Part model, mm, in its own coordinate system. A direction names the side the tool comes from. Round coordinates to 2 decimals unless told otherwise and drop trailing zeros. Loops run counter-clockwise (first coordinate to the right, second up) from the corner with the lowest first, then second, coordinate; pieces in that order, holes last. Notation, with made-up numbers: M 52,22 L 110,22 A24 ccw 110,50 Z; hole C 65,41.25 d5. An arc over 180 degrees is marked long. Put each result on its own line as item: value. Start each with the question number.
```python
from build123d import *
from build123d.topology import SkipClean

# Parameters (mm, degrees)
ESQUISSE1_W                                       = 60.8
ESQUISSE1_H                                       = 121.6
BOSS_EXTRU_1_DEPTH                                = 91.2
ESQUISSE2_W                                       = 60.8
ESQUISSE2_H                                       = 60.8
ENL_V_MAT_EXTRU_1_DEPTH                           = 126.342411019
ESQUISSE3_W                                       = 51.8
ESQUISSE3_H                                       = 51.8
ENL_V_MAT_EXTRU_2_DEPTH                           = 60.8
BOSS_EXTRU_3_DEPTH                                = 4
ESQUISSE6_W                                       = 51.8
ESQUISSE6_H                                       = 51.8
ENL_V_MAT_EXTRU_3_DEPTH                           = 60.8
D_GAGEMENT_1_43_D                                 = 7.14248
FRAISAGE_POUR_VIS_T_TE_FRAIS_E_BOMB_E_D           = 4.3053
FRAISAGE_POUR_VIS_T_TE_FRAIS_E_BOMB_E_DEPTH       = 4.5
FRAISAGE_POUR_VIS_T_TE_FRAIS_E_BOMB_E_CSINK_D     = 7.0866
FRAISAGE_POUR_VIS_T_TE_FRAIS_E_BOMB_E_CSINK_ANGLE = 82
D_GAGEMENT_1_42_D                                 = 7.14248
D_GAGEMENT_1_42_DEPTH                             = 20
BOSS_EXTRU_5_DEPTH                                = 4
CHANFREIN1_SIZE                                   = 4
ESQUISSE26_W                                      = 60.8
ESQUISSE26_H                                      = 60.8
ESQUISSE26_W_2                                    = 51.800000032
ESQUISSE26_H_2                                    = 51.800000032
BOSS_EXTRU_8_DEPTH                                = 60.800000066
ESQUISSE27_R                                      = 3.57124
BOSS_EXTRU_9_DEPTH                                = 1.35


with BuildPart() as part:
    # Esquisse1 → Boss.-Extru.1 (new, symmetric)
    with BuildSketch(Plane.XY):
        Rectangle(ESQUISSE1_W, ESQUISSE1_H)
    extrude(amount=BOSS_EXTRU_1_DEPTH, both=True)

    # Esquisse2 → Enlèv. mat.-Extru.1 (cut, through all)
    with BuildSketch(Plane.ZY.offset(30.4)):
        with Locations((-60.8, 30.4)):
            Rectangle(ESQUISSE2_W, ESQUISSE2_H)
    enl_v_mat_extru_1 = extrude(amount=-ENL_V_MAT_EXTRU_1_DEPTH, mode=Mode.SUBTRACT)

    # Esquisse3 → Enlèv. mat.-Extru.2 (cut)
    with BuildSketch(Plane(origin=(0, 0, -91.2), x_dir=(-1, 0, 0), z_dir=(0, 0, -1))):
        with Locations((0, -30.4)):
            Rectangle(ESQUISSE3_W, ESQUISSE3_H)
    enl_v_mat_extru_2 = extrude(amount=-ENL_V_MAT_EXTRU_2_DEPTH, mode=Mode.SUBTRACT)

    # Symétrie2: Enlèv. mat.-Extru.1, Enlèv. mat.-Extru.2 across plane
    add(enl_v_mat_extru_1.mirror(Plane.XY), mode=Mode.SUBTRACT)
    add(enl_v_mat_extru_2.mirror(Plane.XY), mode=Mode.SUBTRACT)

    # Esquisse10 → Boss.-Extru.3 (add)
    with BuildSketch(Plane(origin=(27.1, 0, 0), x_dir=(0, 0, -1), z_dir=(1, 0, 0))):
        Polygon((30.4, 60.8), (30.4, 0), (91.2, 0), align=None)
        Polygon((-30.4, 60.8), (-91.2, 0), (-30.4, 0), align=None)
    extrude(amount=-BOSS_EXTRU_3_DEPTH)

    # Esquisse6 → Enlèv. mat.-Extru.3 (cut)
    with BuildSketch(Plane(origin=(0, 60.8, 0), x_dir=(1, 0, 0), z_dir=(0, 1, 0))):
        Rectangle(ESQUISSE6_W, ESQUISSE6_H)
    extrude(amount=-ENL_V_MAT_EXTRU_3_DEPTH, mode=Mode.SUBTRACT)

    # Dégagement 1/43 (through all)
    with Locations(Plane(origin=(27.1, 0, 0), x_dir=(0, 0, -1), z_dir=(1, 0, 0))):
        with Locations((45.6, 15.2), (-45.6, 15.2)):
            Hole(D_GAGEMENT_1_43_D / 2)

    # Fraisage pour vis _ t_te frais_e bomb_e
    with Locations(Plane(origin=(30.4, 0, 0), x_dir=(0, 0, -1), z_dir=(1, 0, 0))):
        with Locations((-60.8, -30.4), (0, 30.4), (60.8, -30.4)):
            CounterSinkHole(FRAISAGE_POUR_VIS_T_TE_FRAIS_E_BOMB_E_D / 2, FRAISAGE_POUR_VIS_T_TE_FRAIS_E_BOMB_E_CSINK_D / 2, depth=FRAISAGE_POUR_VIS_T_TE_FRAIS_E_BOMB_E_DEPTH, counter_sink_angle=FRAISAGE_POUR_VIS_T_TE_FRAIS_E_BOMB_E_CSINK_ANGLE)

    # Dégagement 1/42
    with Locations(Plane(origin=(0, -60.8, 0), x_dir=(-1, 0, 0), z_dir=(0, -1, 0))):
        with Locations((0, 78.7), (0, -78.7)):
            Hole(D_GAGEMENT_1_42_D / 2, depth=D_GAGEMENT_1_42_DEPTH)

    # Esquisse23 → Boss.-Extru.5 (add)
    # profile 1 of 2: a face of its own
    with BuildSketch(Plane.ZY.offset(-23.1)):
        Polygon((-41.197704197, 22.825), (-50.002295803, 22.825), (-54.404591605, 15.2), (-50.002295803, 7.575), (-41.197704197, 7.575), (-36.795408395, 15.2), align=None)
        Polygon((-40.25951001, 15.2), (-42.929755005, 19.825), (-48.270244995, 19.825), (-50.94048999, 15.2), (-48.270244995, 10.575), (-42.929755005, 10.575), align=None, mode=Mode.SUBTRACT)
    # profile 2 of 2: a face of its own
    with BuildSketch(Plane.ZY.offset(-23.1)):
        Polygon((54.404591605, 15.2), (50.002295803, 22.825), (41.197704197, 22.825), (36.795408395, 15.2), (41.197704197, 7.575), (50.002295803, 7.575), align=None)
        Polygon((50.94048999, 15.2), (48.270244995, 19.825), (42.929755005, 19.825), (40.25951001, 15.2), (42.929755005, 10.575), (48.270244995, 10.575), align=None, mode=Mode.SUBTRACT)
    extrude(amount=BOSS_EXTRU_5_DEPTH)

    # Chanfrein1
    chanfrein1_edges = [part.edges().sort_by_distance(p)[0] for p in [
        (23.1, 19.0125, 38.996556296),
        (23.1, 11.3875, 38.996556296),
        (23.1, 7.575, 45.6),
        (23.1, 11.3875, 52.203443704),
        (23.1, 19.0125, 52.203443704),
        (23.1, 22.825, 45.6),
        (23.1, 11.3875, -38.996556296),
        (23.1, 19.0125, -38.996556296),
        (23.1, 7.575, -45.6),
        (23.1, 11.3875, -52.203443704),
        (23.1, 22.825, -45.6),
        (23.1, 19.0125, -52.203443704),
    ]]
    chamfer(chanfrein1_edges, length=CHANFREIN1_SIZE - 0.0001)  # a hair under: the kernel refuses the full size

    # Esquisse26 → Boss.-Extru.8 (add)
    with BuildSketch(Plane.ZY.offset(30.4)):
        with Locations((0, -30.4)):
            Rectangle(ESQUISSE26_W, ESQUISSE26_H)
        with Locations((0, -30.4)):
            Rectangle(ESQUISSE26_W_2, ESQUISSE26_H_2, mode=Mode.SUBTRACT)
    extrude(amount=BOSS_EXTRU_8_DEPTH)

    # Esquisse27 → Boss.-Extru.9 (add)
    with SkipClean():  # the faces are left unmerged after this step: merging them gives an invalid solid
        with BuildSketch(Plane.XZ.offset(60.8)):
            Polygon((-30.4, -91.2), (30.4, -91.2), (30.4, 91.2), (-30.4, 91.2), (-30.4, 30.4), (-91.200000066, 30.4), (-91.200000066, -30.4), (-30.4, -30.4), align=None)
            with Locations(Location((0, 78.7, 0), (0, 0, 270))):
                Circle(ESQUISSE27_R, mode=Mode.SUBTRACT)
            with Locations(Location((0, -78.7, 0), (0, 0, 270))):
                Circle(ESQUISSE27_R, mode=Mode.SUBTRACT)
        extrude(amount=BOSS_EXTRU_9_DEPTH)
    add(part.part.scale(1), mode=Mode.REPLACE)  # the faces are merged on a copy


solid = part.part
```
1. Wall check: L1, parallel to Z at x = 0, y = -58; L2, parallel to Z at x = 26.75, y = -30.4; L3, parallel to X at y = -7, z = -63.5. Give the ranges that are in metal, low to high.
2. Which spindle directions (+Z, -Z, +X, -X, +Y, -Y) get a long thin tool onto all of the face, cutting with end or side? Do faces 1 (the flat face through (-30.4, -31, -60)), 2 (the flat face through (0, 31, -25.9)), 3 (the flat face through (19.1, 11.9, -41.8)), 4 (the flat face through (-30.4, -31, 0)). Say none if no direction does.
3. Mould opens along Z. For faces 5 (the flat face through (21.1, 10.5, -54)), 6 (the flat face through (0, -56.3, -61)), 7 (the flat face through (-60, -56.3, 0)) say: released by +Z, released by -Z, zero draft, split by the parting line, or undercut.
4. Cut at D-D, the plane z = 0. Give the cut face in (x, y), and give its area (3 significant figures).
5. Cut at C-C, the plane x = -67. Give the cut face in (y, z).
6. Drop flat-ended pins along their axis: pin 1 (6 mm diameter, centred on x = -9, z = 21.5, fed in from +Y); pin 2 (1.5 mm diameter, centred on x = -29, y = 5, fed in from -Z); pin 3 (2.5 mm diameter, centred on y = 30.4, z = 0, fed in from -X). Give the stop position or say it passes through.
7. Cut at A-A, the plane z = 45.6. Give the number of separate pieces and of enclosed holes in the cut face, and give its area (3 significant figures).
Results list:
1. L1: z = -91.2 to -82.27, -75.13 to 75.13, 82.27 to 91.2
1. L2: z = -91.2 to -62.95, -58.65 to 58.65, 62.95 to 91.2
1. L3: x = -30.4 to -25.9, 25.9 to 30.4
2. face 1: -Z, -X, +Y, -Y
2. face 2: +Y
2. face 3: -Z, -X, +Y
2. face 4: -X
3. face 5: released by -Z
3. face 6: zero draft
3. face 7: undercut
4. outline: M -91.2,-62.15 L 30.4,-62.15 L 30.4,26.86 L 28.8,28.25 L 25.9,28.25 L 25.9,0 L -25.9,0 L -25.9,60.8 L -30.4,60.8 L -30.4,0 L -91.2,0 L -91.2,-4.5 L -30.4,-4.5 L -30.4,-56.3 L -91.2,-56.3 Z; M 25.9,32.55 L 28.8,32.55 L 30.4,33.94 L 30.4,60.8 L 25.9,60.8 Z
4. area: 4,930 mm^2
5. outline: M -62.15,-30.4 L 0,-30.4 L 0,30.4 L -62.15,30.4 Z; hole M -56.3,-25.9 L -4.5,-25.9 L -4.5,25.9 L -56.3,25.9 Z
6. pin 1: stops at y = 0
6. pin 2: stops at z = -30.4
6. pin 3: stops at x = -30.4
7. separate pieces: 2
7. enclosed holes: 1
7. area: 1,290 mm^2
